```python
from build123d import *

# Parameters (mm, degrees)
F1_DEPTH = 19.05
F3_DEPTH = 7.62
F5_DEPTH = 7.62
F6_R     = 3.302
F7_DEPTH = 19.05
F8_R     = 5.08
F9_DEPTH = 16.002


with BuildPart() as f1:
    # F0 (on Right) → F1 (new body)
    with BuildSketch(Plane.YZ):
        with BuildLine():
            Line((215.571838, -73.145718), (215.571838, 77.657629))
            Line((215.571838, 77.657629), (-216.228162, 77.657629))
            Line((-216.228162, 77.657629), (-216.228162, -73.145718))
            ThreePointArc((-216.228162, -73.145718), (-215.497416, -76.929203), (-213.410296, -80.168443))
            Line((-213.410296, -80.168443), (-131.536695, -165.765835))
            Line((-131.536695, -165.765835), (-131.536695, -513.745835))
            Line((-131.536695, -513.745835), (-215.9, -602.645835))
            Line((-215.9, -602.645835), (-215.9, -805.845835))
            Line((-215.9, -805.845835), (-63.5, -805.845835))
            Line((-63.5, -805.845835), (0, -721.487939))
            Line((0, -721.487939), (63.5, -805.845835))
            Line((63.5, -805.845835), (215.9, -805.845835))
            Line((215.9, -805.845835), (215.9, -735.995835))
            Line((215.9, -735.995835), (196.85, -735.995835))
            Line((196.85, -735.995835), (196.85, -634.395835))
            Line((196.85, -634.395835), (215.9, -634.395835))
            Line((215.9, -634.395835), (215.9, -602.645835))
            Line((215.9, -602.645835), (131.536695, -513.745835))
            Line((131.536695, -513.745835), (131.536695, -165.765835))
            Line((131.536695, -165.765835), (212.782136, -80.138879))
            ThreePointArc((212.782136, -80.138879), (214.848676, -76.910248), (215.571838, -73.145718))
        make_face()
    extrude(amount=F1_DEPTH)

    # F2 (on face) → F3 (cut)
    with BuildSketch(Plane.YZ.offset(19.05)):
        Polygon((191.608355, -700.919833), (196.842454, -682.602991), (-145.071934, -584.899811), (-150.306033, -603.216653), align=None)
    extrude(amount=-F3_DEPTH, mode=Mode.SUBTRACT)

    # F4 (on face) → F5 (cut)
    with BuildSketch(Plane.YZ.offset(19.05)):
        Polygon((-216.228162, -71.276438), (216.173725, -71.276438), (215.571838, -52.226438), (-216.228162, -52.226438), align=None)
    extrude(amount=-F5_DEPTH, mode=Mode.SUBTRACT)

    # F6 (on face) → F7 (cut)
    with BuildSketch(Plane.YZ):
        with Locations((-178.128162, -62.640438)):
            Circle(F6_R)
        with Locations((177.471838, -62.640438)):
            Circle(F6_R)
        with Locations((206.427838, 55.305629)):
            Circle(F6_R)
    extrude(amount=F7_DEPTH, mode=Mode.SUBTRACT)

    # F8 (on face) → F9 (cut)
    with BuildSketch(Plane.YZ):
        with Locations((188.722, -723.295835)):
            Circle(F8_R)
        with Locations((188.722, -647.097349)):
            Circle(F8_R)
    extrude(amount=F9_DEPTH, mode=Mode.SUBTRACT)


solid = f1.part
```
CAD build for the part. Positions are in the model's coordinates, mm. A direction names the side the tool comes from. Round coordinates to 2 decimals unless told otherwise and drop trailing zeros. Write each loop counter-clockwise with the first axis right and the second up, starting at its lowest first coordinate (ties: lowest second). Pieces come first, ordered by that corner, then holes. Notation, with made-up numbers: (-8, 8.25) - (-4, 8.25) arc R31 ccw to (-4, 35.25) - close; hole circle Ø6 at (69.25, 54.5). An arc over 180 degrees is marked (long way). Return JSON: item names as keys, results as strings. Group by question number.
Item 1: Band-saw the part on A-A on y = 77. List the corners of the cut face in (x, z), plus the area to 3 significant figures.
Item 2: Probe probe 1 along Z at (x, y) = (17.5, 140.5); probe 2 along Z at (x, y) = (9.5, -179); probe 3 along Z at (x, y) = (12, -145). List the from-to ranges inside material, lowest first.
Item 3: 3-axis set-ups, long thin cutter, end or side, ignore diameter. For faces 1 (the face through (9.392, -173.047, -122.368)), 2 (the face through (11.43, -3, -62)), 3 (the face through (9, 206, -634.396)), 4 (the face through (15.293, 18.258, -651.384)): which of +Z, -Z, +X, -X, +Y, -Y reach the whole face in a straight line?
Item 4: Flat gauge pins, fed straight in: pin 1 Ø5.5 at (x, z) = (13, -678) entering from +Y; pin 2 Ø10 at (x, z) = (3.5, -210) entering from -Y; pin 3 Ø6 at (y, z) = (-178.13, -62.64) entering from +X; pin 4 Ø9 at (y, z) = (188.72, -723.3) entering from -X. Where does each tip first touch, or does it go through?
Item 5: Band-saw the part on C-C on x = 5.5. List the corners of the cut face in (y, z), plus the area to 3 significant figures.
Item 6: Band-saw the part on B-B on z = -409. List the corners of the cut face in (x, y).
Item 7: Band-saw the part on D-D on z = -560. List the corners of the cut face in (x, y), plus the area to 3 significant figures.
Item 8: Mould opens along Z. For faces 5 (the face through (15.293, 28.279, -634.435)), 6 (the face through (9, 215.572, 1)), 7 (the face through (9.39, 31.31, -763.08)) say: +Z half, -Z half, draft (parallel to the pull), parting line (faces both ways), or undercut.
Resolved:
{
 "1": {"outline": "(0, -805.85) - (19.05, -805.85) - (19.05, -668.17) - (11.43, -668.17) - (11.43, -648.36) - (19.05, -648.36) - (19.05, -71.28) - (11.43, -71.28) - (11.43, -52.23) - (19.05, -52.23) - (19.05, 77.66) - (0, 77.66) - close", "area": "16,500 mm²"},
 "2": {"probe 1": "z = -805.85 to -686.32, -666.5 to -523.19, -156.32 to -71.28, -52.23 to 77.66", "probe 2": "z = -805.85 to -563.76, -116.14 to -65.83, -59.46 to 77.66", "probe 3": "z = -805.85 to -604.73, -584.92 to -527.93, -151.69 to -71.28, -52.23 to 77.66"},
 "3": {"face 1": "+X, -X, -Y", "face 2": "+X, +Y, -Y", "face 3": "+X, -X, +Y", "face 4": "+X"},
 "4": {"pin 1": "stops at y = 196.85", "pin 2": "stops at y = -131.54", "pin 3": "passes through", "pin 4": "stops at x = 16"},
 "5": {"outline": "(-216.23, -73.15) arc R10.16 ccw to (-213.41, -80.17) - (-131.54, -165.77) - (-131.54, -513.75) - (-215.9, -602.65) - (-215.9, -805.85) - (-63.5, -805.85) - (0, -721.49) - (63.5, -805.85) - (215.9, -805.85) - (215.9, -736) - (196.85, -736) - (196.85, -634.4) - (215.9, -634.4) - (215.9, -602.65) - (131.54, -513.75) - (131.54, -165.77) - (212.78, -80.14) arc R10.16 ccw to (215.57, -73.15) - (215.57, 77.66) - (-216.23, 77.66) - close; hole circle Ø6.6 at (-178.13, -62.64); hole circle Ø6.6 at (177.47, -62.64); hole circle Ø10.16 at (188.72, -723.3); hole circle Ø10.16 at (188.72, -647.1); hole circle Ø6.6 at (206.43, 55.31)", "area": "300,000 mm²"},
 "6": {"outline": "(0, -131.54) - (19.05, -131.54) - (19.05, 131.54) - (0, 131.54) - close"},
 "7": {"outline": "(0, -175.43) - (19.05, -175.43) - (19.05, 175.43) - (0, 175.43) - close", "area": "6,680 mm²"},
 "8": {"face 5": "undercut", "face 6": "draft", "face 7": "-Z half"}
}
